```python
from build123d import *

# Parameters (mm, degrees)
SKETCH1_R                = 45.5
SKETCH1_R_2              = 42.5
BOSS_EXTRUDE1_DEPTH      = 30
SKETCH2_R                = 45.5
BOSS_EXTRUDE2_DEPTH      = 2
SKETCH3_R                = 7
CUT_EXTRUDE1_DEPTH       = 2
SKETCH7_W                = 3
SKETCH7_H                = 10
BOSS_EXTRUDE4_DEPTH      = 26
BOSS_EXTRUDE4_DEPTH_BACK = 2
SKETCH8_R                = 19.890165718
SKETCH8_R_2              = 18.390165718
BOSS_EXTRUDE5_DEPTH      = 1
CUT_EXTRUDE4_DEPTH       = 5.5
CUT_EXTRUDE5_DEPTH       = 58.5
CUT_EXTRUDE6_DEPTH       = 1


with BuildPart() as part:
    # Sketch1 → Boss-Extrude1 (new body)
    with BuildSketch(Plane(origin=(0, 0, 0), x_dir=(1, 0, 0), z_dir=(0, 1, 0))):
        Circle(SKETCH1_R)
        Circle(SKETCH1_R_2, mode=Mode.SUBTRACT)
    extrude(amount=BOSS_EXTRUDE1_DEPTH)

    # Sketch2 → Boss-Extrude2 (add)
    with BuildSketch(Plane.XZ):
        Circle(SKETCH2_R)
    extrude(amount=-BOSS_EXTRUDE2_DEPTH)

    # Sketch3 → Cut-Extrude1 (cut)
    with BuildSketch(Plane(origin=(0, 2, 0), x_dir=(1, 0, 0), z_dir=(0, 1, 0))):
        Circle(SKETCH3_R)
    extrude(amount=-CUT_EXTRUDE1_DEPTH, mode=Mode.SUBTRACT)

    # Sketch7 → Boss-Extrude4 (add, two sides)
    with BuildSketch(Plane(origin=(0, 2, 0), x_dir=(1, 0, 0), z_dir=(0, 1, 0))) as boss_extrude4_sk:
        with Locations((0, 47.473521163)):
            Rectangle(SKETCH7_W, SKETCH7_H)
        Polygon((46.193402353, 24.937722476), (37.533148315, 19.937722476), (36.033148315, 22.535798687), (44.693402353, 27.535798687), align=None)
    extrude(amount=BOSS_EXTRUDE4_DEPTH)
    extrude(boss_extrude4_sk.sketch, amount=-BOSS_EXTRUDE4_DEPTH_BACK)

    # Sketch8 → Boss-Extrude5 (add)
    with BuildSketch(Plane(origin=(0, 2, 0), x_dir=(1, 0, 0), z_dir=(0, 1, 0))):
        Circle(SKETCH8_R)
        Circle(SKETCH8_R_2, mode=Mode.SUBTRACT)
    extrude(amount=BOSS_EXTRUDE5_DEPTH)

    # Sketch10 → Cut-Extrude4 (cut)
    with BuildSketch(Plane.XZ):
        Polygon((2.016687189, -18.494703278), (14.981867268, -10.951222284), (10.958677405, -4.036459575), (-2.006502675, -11.579940569), align=None)
    extrude(amount=-CUT_EXTRUDE4_DEPTH, mode=Mode.SUBTRACT)

    # Sketch11 → Cut-Extrude5 (cut)
    with BuildSketch(Plane(origin=(0, 2, 0), x_dir=(1, 0, 0), z_dir=(0, 1, 0))):
        Polygon((-32.606600292, -26.874098434), (-35.165226496, -28.87311631), (-33.824988888, -37.754161376), (-11.7382848, -48.772412552), (-7.925983096, -44.804338986), (-7.495155029, -41.738838001), (-9.978475631, -35.419229659), (-25.965270809, -26.874098434), align=None)
    extrude(amount=CUT_EXTRUDE5_DEPTH, mode=Mode.SUBTRACT)

    # Sketch12 → Cut-Extrude6 (cut)
    with BuildSketch(Plane.XZ):
        Polygon((-6.912265346, 1.104802147), (-24.20763883, -9.480307189), (-19.814483018, -16.658435267), (-2.519109534, -6.073325931), align=None)
    extrude(amount=-CUT_EXTRUDE6_DEPTH, mode=Mode.SUBTRACT)


solid = part.part
```
Source: CAD feature listing. Evaluate the final solid. Frame: model axes, mm. A direction names the side the tool comes from. Coordinates: 2 decimals unless noted, no trailing zeros. Order: outer loops, then holes, each group sorted by start corner. A loop starts at its lowest first (then second) coordinate and runs counter-clockwise, first axis right, second up. Notation, with made-up numbers: (77, 68) - (89, 68) arc R12 cw to (89, 86) - close; hole circle Ø7 at (86, -11.75). An arc over 180 degrees is marked (long way). One line per item, written item: value.
1) Cut plane B-B on y = 14.75. Output: boundary loops of the cut face in (x, z).
Computed values:
outline: (-35.17, 28.87) arc R45.5 ccw to (-1.5, -45.48) - (-1.5, -52.47) - (1.5, -52.47) - (1.5, -45.48) arc R45.5 ccw to (38.63, -24.04) - (44.69, -27.54) - (46.19, -24.94) - (40.13, -21.44) arc R45.5 ccw to (-7.93, 44.8) - (-7.51, 41.83) arc R42.5 cw to (37.53, -19.94) - (36.03, -22.54) arc R42.5 cw to (1.5, -42.47) - (-1.5, -42.47) arc R42.5 cw to (-32.8, 27.03) - close
2) Ray query, line 1 (X direction, y = 2.4, z = 0); line 2 (Z direction, x = 0, y = 2.7); line 3 (Z direction, x = 0, y = 1.25). Return the intervals inside material, ascending. Write a range as [from, to].
Computed values:
line 1: x = [-45.5, -42.5], [-19.89, -18.39], [18.39, 19.89], [42.5, 45.5]
line 2: z = [-52.47, -42.47], [-19.89, -18.39], [18.39, 19.89], [42.5, 45.5]
line 3: z = [-52.47, -15.03], [-10.41, -7], [7, 45.5]
3) Cut plane D-D on z = 12. Output: boundary loops of the cut face in (x, y).
Computed values:
outline: (-43.89, 0) - (43.89, 0) - (43.89, 30) - (40.77, 30) - (40.77, 2) - (15.86, 2) - (15.86, 3) - (13.94, 3) - (13.94, 2) - (-13.94, 2) - (-13.94, 3) - (-15.86, 3) - (-15.86, 2) - (-40.77, 2) - (-40.77, 30) - (-43.89, 30) - close
4) Mould query, pull axis X, two halves, no side actions, for faces 6 (the face through (43.205, 14.196, -23.213)), 7 (the face through (36.794, 14.818, -21.219)), 8 (the face through (-11.505, 0.493, -11.573)), 9 (the face through (10, 0, -4)). Classes: released by +X, released by -X, zero draft, split by the parting line, or undercut.
Computed values:
face 6: released by +X
face 7: undercut
face 8: undercut
face 9: zero draft
5) Reachability of faces 1 (the face through (-22.04, 0.49, -13.02)), 2 (the face through (42, 28, -25)), 3 (the face through (8.409, 0.812, -14.776)), 4 (the face through (9.34, 2.49, -15.84)), 5 (the face through (1.5, 14, -49)) from +Z, -Z, +X, -X, +Y, -Y: full face, straight path, thin tool, end or side. Return the list, or none.
Computed values:
face 1: -Y
face 2: -Z, +X, +Y
face 3: +Y, -Y
face 4: +Y
face 5: -Z, +X, +Y, -Y
6) Cut plane A-A on z = 0. Output: boundary loops of the cut face in (x, y), plus the area to 3 significant figures.
Computed values:
outline: (-45.5, 0) - (-8.72, 0) - (-8.72, 1) - (-7, 1) - (-7, 2) - (-18.39, 2) - (-18.39, 3) - (-19.89, 3) - (-19.89, 2) - (-42.5, 2) - (-42.5, 30) - (-45.5, 30) - close; (7, 0) - (45.5, 0) - (45.5, 30) - (42.5, 30) - (42.5, 2) - (19.89, 2) - (19.89, 3) - (18.39, 3) - (18.39, 2) - (7, 2) - close
area: 323 mm^2
7) Cut plane C-C on x = 0. State how many separate pieces and enclosed holes the cut face has, plus the area to 3 significant figures.
Computed values:
separate pieces: 3
enclosed holes: 0
area: 512 mm^2
8) Contact query for flat-ended pins moving along their axis: pin 1 (3 mm diameter, centred on x = -6, z = 34.5, fed in from -Y); pin 2 (18 mm diameter, centred on x = 0, z = 0, fed in from +Y); pin 3 (1.8 mm diameter, centred on x = 42, z = -24.5, fed in from +Y); pin 4 (3.5 mm diameter, centred on x = 9.5, z = -15, fed in from +Y). Output: stop coordinate, or through.
Computed values:
pin 1: stops at y = 0
pin 2: stops at y = 2
pin 3: stops at y = 28
pin 4: stops at y = 3
